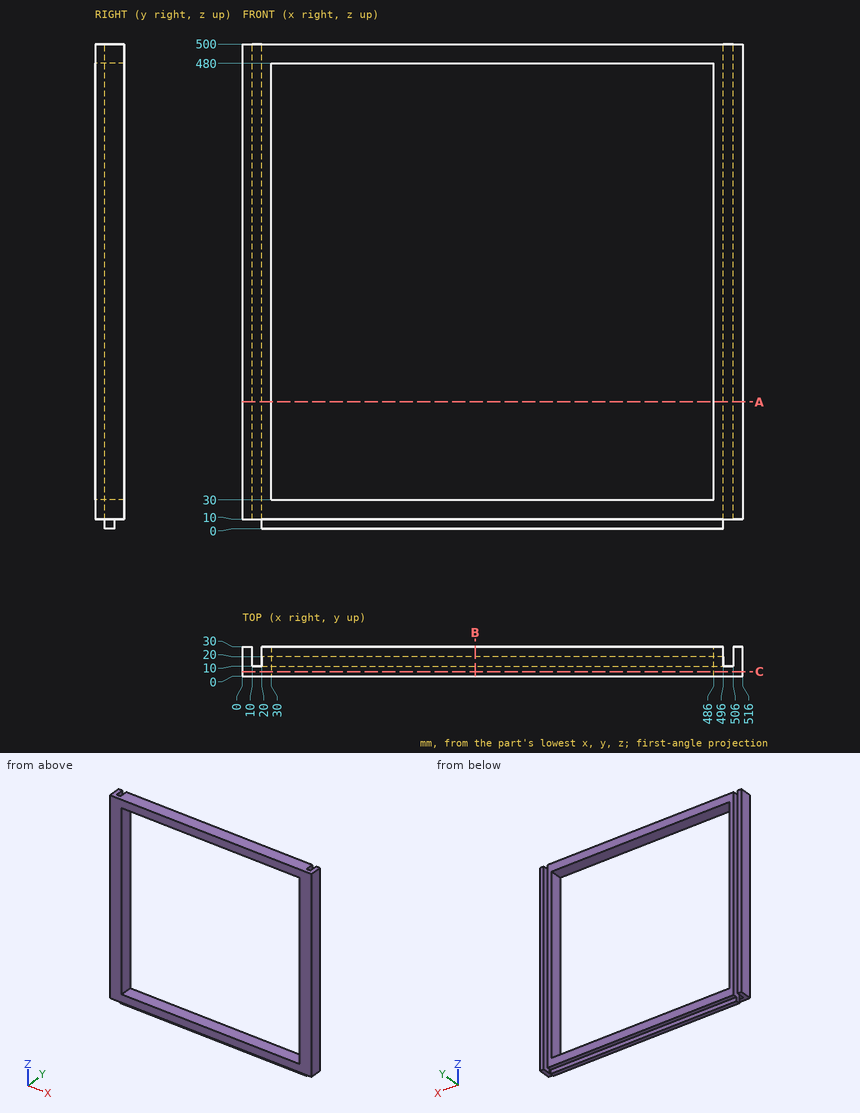
Input: dimensioned drawing with shaded views. Units: mm. Origin: part minimum x, y, z. Give positions to 0.01 mm unless a question says otherwise; leave off trailing zeros. Loops run counter-clockwise (first coordinate to the right, second up) from the corner with the lowest first, then second, coordinate; pieces in that order, holes last. Notation, with made-up numbers: M -23.5,39.25 L 15.5,39.25 A20 ccw 15.5,74.25 Z; hole C 67,69.5 d8. An arc over 180 degrees is marked long. Put each result on its own line as item: value. Start each with the question number.
1) Cut plane B-B (x = 240). Output: boundary loops of the cut face in (y, z), then the cut area to 3 significant figures.
2) Cut plane A-A (z = 131). Output: boundary loops of the cut face in (x, y), then the cut area to 3 significant figures.
3) Contact query for flat-ended pins moving along their axis: pin 1 (3 mm diameter, centred on x = 156.5, y = 27, fed in from -Z); pin 2 (5 mm diameter, centred on x = 201.5, z = 4, fed in from +Y); pin 3 (3 mm diameter, centred on x = 14, z = 340.5, fed in from +Y). Output: stop coordinate, or through.
4) Ray query, line 1 along X through (y, z) = (28.25, 136); line 2 along Z through (x, y) = (229, 22.5); line 3 along X through (y, z) = (2.75, 254.5). Return the intervals inside material, ascending.
5) Cut plane C-C (y = 4.5). Output: boundary loops of the cut face in (x, z), then the cut area to 3 significant figures.
Verdict:
1. outline: M 0,10 L 10,10 L 10,0 L 20,0 L 20,10 L 30,10 L 30,30 L 0,30 Z; M 0,480 L 30,480 L 30,500 L 0,500 Z
1. area: 1,300 mm2
2. outline: M 0,0 L 30,0 L 30,30 L 20,30 L 20,10 L 10,10 L 10,30 L 0,30 Z; M 486,0 L 516,0 L 516,30 L 506,30 L 506,10 L 496,10 L 496,30 L 486,30 Z
2. area: 1,400 mm2
3. pin 1: z = 10
3. pin 2: y = 20
3. pin 3: y = 10
4. line 1: 0 to 10, 20 to 30, 486 to 496, 506 to 516
4. line 2: 10 to 30, 480 to 500
4. line 3: 0 to 30, 486 to 516
5. outline: M 0,10 L 516,10 L 516,500 L 0,500 Z; hole M 30,30 L 486,30 L 486,480 L 30,480 Z
5. area: 47,600 mm2
